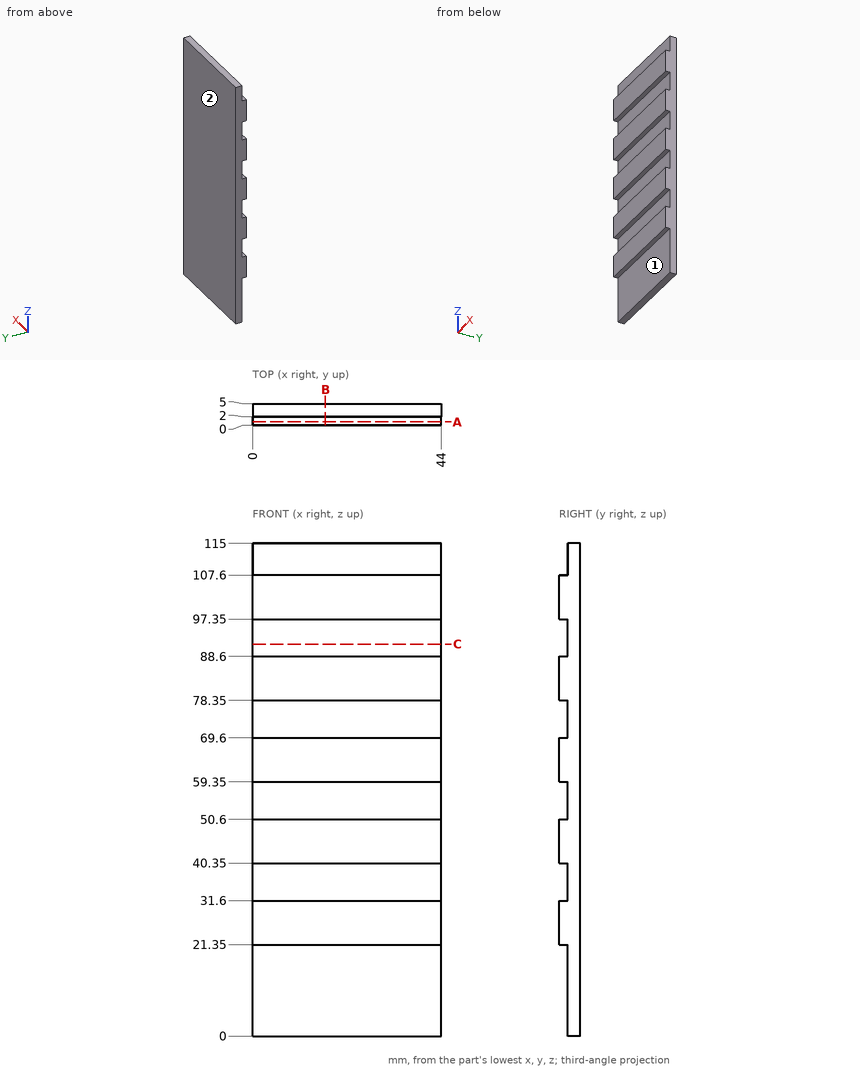
Drawing for the job (mm, zero at the part's lowest x, y, z). A direction names the side the tool comes from. Give positions to 0.01 mm unless a question says otherwise; leave off trailing zeros. Order: outer loops, then holes, each group sorted by start corner. A loop starts at its lowest first (then second) coordinate and runs counter-clockwise, first axis right, second up. Notation, with made-up numbers: M -16.5,49 L 8.5,49 A30 cw 8.5,81 Z; hole C -5.75,20.5 d1. An arc over 180 degrees is marked long. Write item = value, one per line. Start each with the question number.
(1) Which spindle directions (+Z, -Z, +X, -X, +Y, -Y) get a long thin tool onto all of the face, cutting with end or side? Do the marked faces 1 and 2. Say none if no direction does.
(2) Slice it at A-A on y = 0.8. Write the cut outline in (x, z).
(3) Probe L1, parallel to Z at x = 41, y = 0.3; L2, parallel to Y at x = 4, z = 94.5. List the from-to ranges inside material, lowest first. Write a range as [from, to].
(4) Slice it at C-C on z = 91.5. Write the cut outline in (x, y), plus the area to 3 significant figures.
(5) Pin check, flat tips, straight feed: pin 1 Ø2.5 at (x, z) = (11.5, 74) entering from -Y; pin 2 Ø2 at (y, z) = (4.5, 101.5) entering from -X; pin 3 Ø1 at (x, y) = (12.5, 1) entering from -Z. Stop position of each tip, or through.
(6) Slice it at B-B on x = 17. Write the cut outline in (y, z), plus the area to 4 significant figures.
Responses:
q1.face_1 = -Z, +X, -X, -Y
q1.face_2 = +Z, -Z, +X, -X, +Y
q2.outline = M 0,21.35 L 44,21.35 L 44,31.6 L 0,31.6 Z; M 0,40.35 L 44,40.35 L 44,50.6 L 0,50.6 Z; M 0,59.35 L 44,59.35 L 44,69.6 L 0,69.6 Z; M 0,78.35 L 44,78.35 L 44,88.6 L 0,88.6 Z; M 0,97.35 L 44,97.35 L 44,107.6 L 0,107.6 Z
q3.L1 = [21.35, 31.6], [40.35, 50.6], [59.35, 69.6], [78.35, 88.6], [97.35, 107.6]
q3.L2 = [2, 5]
q4.outline = M 0,2 L 44,2 L 44,5 L 0,5 Z
q4.area = 132 mm2
q5.pin_1 = 2
q5.pin_2 = 0
q5.pin_3 = 21.35
q6.outline = M 0,21.35 L 2,21.35 L 2,0 L 5,0 L 5,115 L 2,115 L 2,107.6 L 0,107.6 L 0,97.35 L 2,97.35 L 2,88.6 L 0,88.6 L 0,78.35 L 2,78.35 L 2,69.6 L 0,69.6 L 0,59.35 L 2,59.35 L 2,50.6 L 0,50.6 L 0,40.35 L 2,40.35 L 2,31.6 L 0,31.6 Z
q6.area = 447.5 mm2
